Job drawing, mm, ordinate dimensions from the low corner. One solid piece. Round coordinates to 2 decimals unless told otherwise and drop trailing zeros. Loops run counter-clockwise (first coordinate to the right, second up) from the corner with the lowest first, then second, coordinate; pieces in that order, holes last.
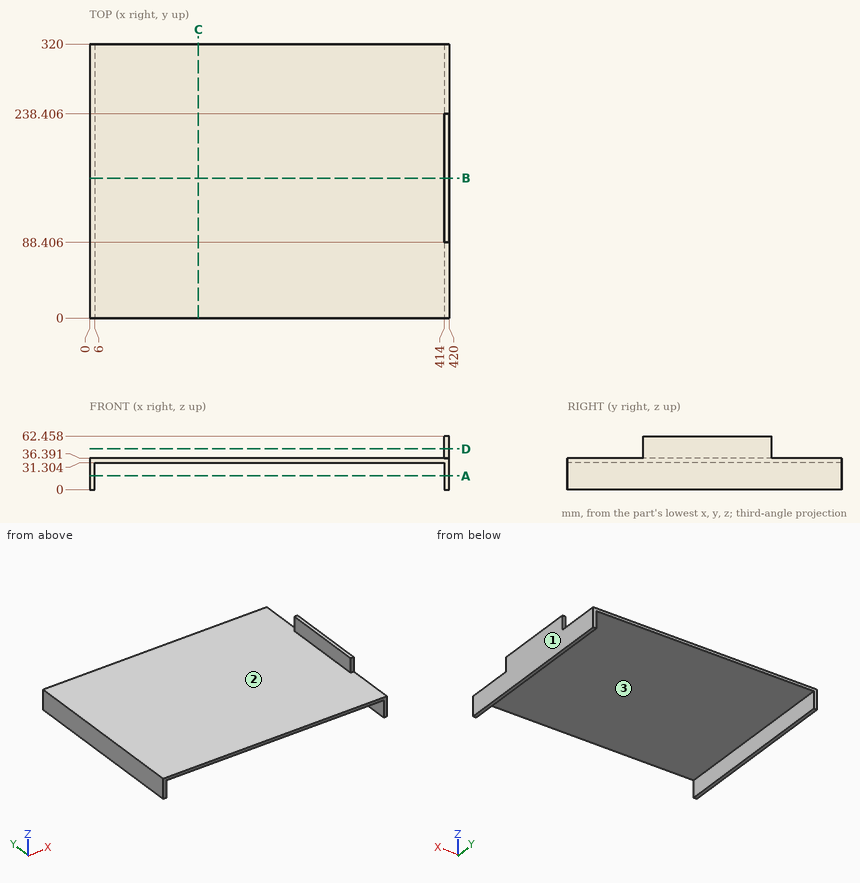
Item 1: Cut at B-B, the plane y = 163.5. Give the cut face in (x, z), plus the area to 3 significant figures.
Answers follow:
outline: (0, 0) - (6, 0) - (6, 31.3) - (414, 31.3) - (414, 0) - (420, 0) - (420, 62.46) - (414, 62.46) - (414, 36.39) - (0, 36.39) - close
area: 2,670 mm2
Item 2: Flat gauge pins, fed straight in: P1, Ø25, axis at y = 138, z = 17.5, coming from the -X side; P2, Ø10, axis at x = 83, y = 258.5, coming from the +Z side; P3, Ø5, axis at x = 416.5, z = 48.5, coming from the +Y side; P4, Ø4, axis at x = 359, y = 250, coming from the -Z side. Where does each tip first touch, or does it go through?
Answers follow:
P1: stops at x = 0
P2: stops at z = 36.39
P3: stops at y = 238.41
P4: stops at z = 31.3
Item 3: Cut at C-C, the plane x = 127. Give the cut face in (y, z).
Answers follow:
outline: (0, 31.3) - (320, 31.3) - (320, 36.39) - (0, 36.39) - close
Item 4: Probe line 1 (X direction, y = 147, z = 16); line 2 (Z direction, x = 295, y = 80.5); line 3 (X direction, y = 93.5, z = 38.5). List the from-to ranges inside material, lowest first.
Answers follow:
line 1: x = 0 to 6, 414 to 420
line 2: z = 31.3 to 36.39
line 3: x = 414 to 420
Item 5: Cut at D-D, the plane z = 47.5. Give the cut face in (x, y).
Answers follow:
outline: (414, 88.41) - (420, 88.41) - (420, 238.41) - (414, 238.41) - close
Item 6: Cut at A-A, the plane z = 16. Give the cut face in (x, y), plus the area to 3 significant figures.
Answers follow:
outline: (0, 0) - (6, 0) - (6, 320) - (0, 320) - close; (414, 0) - (420, 0) - (420, 320) - (414, 320) - close
area: 3,840 mm2
Item 7: Two-plate mould, pull along X, no slides. Class the marked faces 1, 2 and 3: released by +X, released by -X, zero draft, split by the parting line, or undercut.
Answers follow:
face 1: released by +X
face 2: zero draft
face 3: undercut
